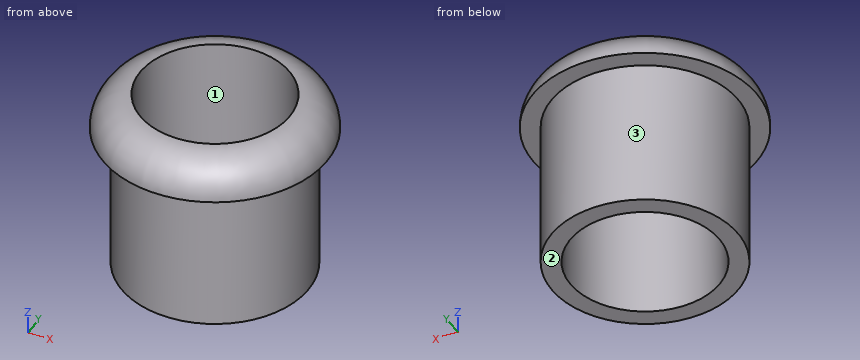
Autodesk Inventor part; units mm, degrees
ref_plane "YZ Plane" through (0, 0, 0) normal (1, 0, 0) x (0, 1, 0)
ref_plane "XZ Plane" through (0, 0, 0) normal (0, 1, 0) x (-1, 0, 0)
ref_plane "XY Plane" through (0, 0, 0) normal (0, 0, 1) x (1, 0, 0)
sketch "Эскиз1" plane through (0, 0, 0) normal (0, 0, 1) x (1, 0, 0)
  circle A0 centre (0, 0) radius 4
  circle A1 centre (0, 0) radius 5
  dimension "d0" = 8
  dimension "d1" = 10
extrude "Выдавливание1" add sketch "Эскиз1" along normal blind 10
sketch "Эскиз2" plane through (0, 0, 10) normal (0, 0, 1) x (1, 0, 0)
  circle A0 centre (0, 0) radius 6
  circle A1 centre (0, 0) radius 5
  dimension "d4" = 12
extrude "Выдавливание2" add sketch "Эскиз2" against normal blind 2
fillet "Сопряжение1" radius 2 1 edges at (-6, 0, 10)
properties part number "hole_big" material "Латунь"
Geometry: final body of the model. Coordinates: model frame, mm. Face numbers are marked on the shaded views. Give positions to 0.01 mm unless a question says otherwise; leave off trailing zeros. Loops run counter-clockwise (first coordinate to the right, second up) from the corner with the lowest first, then second, coordinate; pieces in that order, holes last. Notation, with made-up numbers: M -34,15.25 L 11,15.25 A12 ccw 11,38.25 Z; hole C 70,49.25 d6. An arc over 180 degrees is marked long. Put each result on its own line as item: value. Start each with the question number.
1) Cut plane C-C (z = 2). Output: boundary loops of the cut face in (x, y), then the cut area to 3 significant figures.
2) Contact query for flat-ended pins moving along their axis: pin 1 (4 mm diameter, centred on y = -0.5, z = 5.5, fed in from -X); pin 2 (4 mm diameter, centred on y = -4, z = 1.5, fed in from -X); pin 3 (5 mm diameter, centred on x = -4, z = 5, fed in from -Y). Output: stop coordinate, or through.
3) Ray query, line 1 along X through (y, z) = (-2.75, 8.25); line 2 along Y through (x, z) = (0, 8.25); line 3 along Y through (x, z) = (0, 6.25). Return the intervals inside material, ascending.
4) Pull-direction query (Y, two-part tool) for the marked faces 1, 2 and 3; classes: pulls with the +Y half, pulls with the -Y half, needs draft (parallel to the pull), parting line crosses it, or undercut.
5) Cut plane D-D (z = 8.5). Output: boundary loops of the cut face in (x, y).
Verdict:
1. outline: C 0,0 d10; hole C 0,0 d8
1. area: 28.3 mm2
2. pin 1: x = -5
2. pin 2: x = -4.58
2. pin 3: y = -4.77
3. line 1: -5.32 to -2.9, 2.9 to 5.32
3. line 2: -5.98 to -4, 4 to 5.98
3. line 3: -5 to -4, 4 to 5
4. face 1: undercut
4. face 2: needs draft
4. face 3: parting line crosses it
5. outline: C 0,0 d11.87; hole C 0,0 d8
